```python
from build123d import *

# Parameters (mm, degrees)
SKETCH1_R               = 2
FORMA_B_SICA_DEPTH      = 5
FORMA_B_SICA_2_DEPTH    = 5
BOSS_EXTRUDE2_DEPTH     = 23.3
CARRIL_CREMALLERA_DEPTH = 56.7
ELIMINAR_FILETE_DEPTH   = 23.3
FILLET2_R               = 2


with BuildPart() as part:
    # Sketch1 → Forma básica (new body)
    with BuildSketch(Plane.XY):
        with BuildLine():
            ThreePointArc((-25.85, -9.9), (-27.617766953, -9.167766953), (-28.35, -7.4))
            Line((-28.35, -7.4), (-28.35, 9.9))
            Line((-28.35, 9.9), (-20.15, 9.9))
            Line((-20.15, 9.9), (-20.15, -9.9))
            Line((-20.15, -9.9), (-25.85, -9.9))
        make_face()
        with Locations((-24.25, -5)):
            Circle(SKETCH1_R, mode=Mode.SUBTRACT)
        with Locations((-24.25, 5)):
            Circle(SKETCH1_R, mode=Mode.SUBTRACT)
    extrude(amount=FORMA_B_SICA_DEPTH)



with BuildPart() as body_2:
    # Sketch1 → Forma b_sica 2 (new body)
    with BuildSketch(Plane.XY):
        with BuildLine():
            ThreePointArc((28.35, -7.4), (27.617766953, -9.167766953), (25.85, -9.9))
            Line((25.85, -9.9), (20.15, -9.9))
            Line((20.15, -9.9), (20.15, 9.9))
            Line((20.15, 9.9), (28.35, 9.9))
            Line((28.35, 9.9), (28.35, -7.4))
        make_face()
        with Locations((24.25, 5)):
            Circle(SKETCH1_R, mode=Mode.SUBTRACT)
        with Locations((24.25, -5)):
            Circle(SKETCH1_R, mode=Mode.SUBTRACT)
    extrude(amount=FORMA_B_SICA_2_DEPTH)


with BuildPart() as part_1:
    add(part.part)

    add(body_2.part)  # Boss-Extrude2 merges body 2
    # Sketch1<3> → Boss-Extrude2 (add)
    with BuildSketch(Plane.XY):
        with BuildLine():
            Line((-28.35, 9.9), (-20.15, 9.9))
            Line((-20.15, 9.9), (20.15, 9.9))
            Line((20.15, 9.9), (28.35, 9.9))
            Line((28.35, 9.9), (28.35, 17.4))
            ThreePointArc((28.35, 17.4), (27.617766953, 19.167766953), (25.85, 19.9))
            Line((25.85, 19.9), (-25.85, 19.9))
            ThreePointArc((-25.85, 19.9), (-27.617766953, 19.167766953), (-28.35, 17.4))
            Line((-28.35, 17.4), (-28.35, 9.9))
        make_face()
    extrude(amount=BOSS_EXTRUDE2_DEPTH)

    # Sketch2 → Carril cremallera (add)
    with BuildSketch(Plane(origin=(28.35, 0, 0), x_dir=(0, 0, -1), z_dir=(1, 0, 0))):
        Polygon((-23.3, 19.9), (-19.764466094, 23.435533906), (-19.764466094, 28.435533906), (-35.834466094, 28.435533906), (-35.834466094, 23.435533906), (-32.298932188, 19.9), (-40.298932188, 19.9), (-40.298932188, 33.9), (-15.3, 33.9), (-15.3, 19.9), align=None)
    extrude(amount=-CARRIL_CREMALLERA_DEPTH)

    # Sketch3 → Eliminar filete (add)
    with BuildSketch(Plane.XY.offset(23.3)):
        with BuildLine():
            Line((-28.35, 17.4), (-28.35, 19.9))
            Line((-28.35, 19.9), (-25.85, 19.9))
            ThreePointArc((-25.85, 19.9), (-27.617766953, 19.167766953), (-28.35, 17.4))
        make_face()
        with BuildLine():
            Line((28.35, 19.9), (25.85, 19.9))
            ThreePointArc((25.85, 19.9), (27.617766953, 19.167766953), (28.35, 17.4))
            Line((28.35, 17.4), (28.35, 19.9))
        make_face()
    extrude(amount=-ELIMINAR_FILETE_DEPTH)

    # Fillet2
    fillet2_edges = [part_1.edges().sort_by_distance(p)[0] for p in [
        (28.35, 33.9, 27.799466094),
        (-28.35, 33.9, 27.799466094),
        (-28.35, 19.9, 7.65),
        (28.35, 19.9, 7.65),
    ]]
    fillet(fillet2_edges, radius=FILLET2_R)


solid = part_1.part
```
Check sheet for the modelled part. Datum: model origin and axes. Units: mm. A direction names the side the tool comes from. Give positions to 0.01 mm unless a question says otherwise; leave off trailing zeros. Write each loop counter-clockwise with the first axis right and the second up, starting at its lowest first coordinate (ties: lowest second). Pieces come first, ordered by that corner, then holes.
Item 1: Scan lines: L1, parallel to Y at x = -24.25, z = 2.05; L2, parallel to Z at x = -9.5, y = 24; L3, parallel to Y at x = 15.5, z = 17.5. Record each from-to range of solid material in increasing order.
Item 2: Access from +Z, -Z, +X, -X, +Y, -Y to the whole of each face (thin tool, end or side, straight path). Record for faces 1 (the face through (-20.15, 0, 2)), 2 (the face through (0, 28.436, 28)), 3 (the face through (0, 15, 23.3)), 4 (the face through (-27.78, 19.3, 7.54)).
Item 3: Cross-section at B-B (y = 5). Enter the section's corners in (x, z), and give its area (3 significant figures).
Item 4: Gauge pin test, flat ends, axial feed: pin 1 (9 mm diameter, centred on x = -23.5, y = -5, fed in from +Z); pin 2 (2.5 mm diameter, centred on x = -1.5, z = 34.5, fed in from -Y); pin 3 (17 mm diameter, centred on x = -1, z = 5.5, fed in from +Y). Record the tip position at first contact, or that the pin passes through.
Item 5: Cross-section at D-D (z = 25.5). Enter the section's corners in (x, y), and give its area (3 significant figures).
Item 6: Cross-section at C-C (y = 25). Enter the section's corners in (x, z), and give its area (3 significant figures).
Item 7: Cross-section at A-A (x = -24.25). Enter the section's corners in (y, z).
Item 8: Draft check along Z on faces 5 (the face through (-27.598, -9.187, 2.465)), 6 (the face through (-24, 0, 5)), 7 (the face through (0, 26, 35.834)). Enter one of: released by +Z, released by -Z, zero draft, split by the parting line, or undercut.
Report:
1. L1: y = -9.9 to -7, -3 to 3, 7 to 19.9
1. L2: z = 15.3 to 19.76, 35.83 to 40.3
1. L3: y = 9.9 to 33.9
2. face 1: +Z, -Z, -Y
2. face 2: +X, -X
2. face 3: +Z, +X, -X, -Y
2. face 4: -Z, -X, +Y
3. outline: (-28.35, 0) - (-26.25, 0) - (-26.25, 5) - (-28.35, 5) - close; (-22.25, 0) - (-20.15, 0) - (-20.15, 5) - (-22.25, 5) - close; (20.15, 0) - (22.25, 0) - (22.25, 5) - (20.15, 5) - close; (26.25, 0) - (28.35, 0) - (28.35, 5) - (26.25, 5) - close
3. area: 42.0 mm2
4. pin 1: stops at z = 5
4. pin 2: stops at y = 19.9
4. pin 3: stops at y = 19.9
5. outline: (-28.35, 28.44) - (28.35, 28.44) - (28.35, 31.9) arc R2 ccw to (26.35, 33.9) - (-26.35, 33.9) arc R2 ccw to (-28.35, 31.9) - close
5. area: 308 mm2
6. outline: (-28.35, 15.3) - (28.35, 15.3) - (28.35, 19.76) - (-28.35, 19.76) - close; (-28.35, 35.83) - (28.35, 35.83) - (28.35, 40.3) - (-28.35, 40.3) - close
6. area: 506 mm2
7. outline: (-9.9, 0) - (-7, 0) - (-7, 5) - (-9.9, 5) - close; (-3, 0) - (3, 0) - (3, 5) - (-3, 5) - close; (7, 0) - (19.9, 0) - (19.9, 15.3) - (33.9, 15.3) - (33.9, 40.3) - (19.9, 40.3) - (19.9, 32.3) - (23.44, 35.83) - (28.44, 35.83) - (28.44, 19.76) - (23.44, 19.76) - (19.9, 23.3) - (9.9, 23.3) - (9.9, 5) - (7, 5) - close
8. face 5: zero draft
8. face 6: released by +Z
8. face 7: undercut
